The model under review builds one solid part; all positions refer to its coordinate system, in mm. A direction names the side the tool comes from. Give positions to 0.01 mm unless a question says otherwise; leave off trailing zeros. Write each loop counter-clockwise with the first axis right and the second up, starting at its lowest first coordinate (ties: lowest second). Pieces come first, ordered by that corner, then holes. Notation, with made-up numbers: (50.5, 89) - (93.5, 89) arc R15 cw to (93.5, 107) - close; hole circle Ø11 at (67, 67). An arc over 180 degrees is marked (long way). Write item = value, one per line.
```python
from build123d import *

# Parameters (mm, degrees)
EXTRUDE_1_DEPTH = 5


with BuildPart() as part:
    # 草图1 → 凸台-拉伸1 (new body)
    with BuildSketch(Plane.XY):
        with BuildLine():
            Line((36.5, -9.5), (36.5, 9.5))
            ThreePointArc((36.5, 9.5), (35.621320344, 11.621320344), (33.5, 12.5))
            Line((33.5, 12.5), (-33.5, 12.5))
            ThreePointArc((-33.5, 12.5), (-35.621320344, 11.621320344), (-36.5, 9.5))
            Line((-36.5, 9.5), (-36.5, -9.5))
            ThreePointArc((-36.5, -9.5), (-35.621320344, -11.621320344), (-33.5, -12.5))
            Line((-33.5, -12.5), (-2.5, -12.5))
            Line((-2.5, -12.5), (-2.5, 2.5))
            Line((-2.5, 2.5), (2.5, 2.5))
            Line((2.5, 2.5), (2.5, -12.5))
            Line((2.5, -12.5), (33.5, -12.5))
            ThreePointArc((33.5, -12.5), (35.621320344, -11.621320344), (36.5, -9.5))
        make_face()
        with BuildLine():
            Line((-19.75, -2.5), (-19.75, 6))
            ThreePointArc((-19.75, 6), (-16.5, 9.25), (-13.25, 6))
            Line((-13.25, 6), (-13.25, -2.5))
            ThreePointArc((-13.25, -2.5), (-16.5, -5.75), (-19.75, -2.5))
        make_face(mode=Mode.SUBTRACT)
        with BuildLine():
            Line((19.75, -2.5), (19.75, 6))
            ThreePointArc((19.75, 6), (16.5, 9.25), (13.25, 6))
            Line((13.25, 6), (13.25, -2.5))
            ThreePointArc((13.25, -2.5), (16.5, -5.75), (19.75, -2.5))
        make_face(mode=Mode.SUBTRACT)
    extrude(amount=EXTRUDE_1_DEPTH)


solid = part.part
```
1. Take a section at A-A on x = -16.5. Give the boundary of the cut face in (y, z), and give its area (3 significant figures).
Findings below:
outline = (-12.5, 0) - (-5.75, 0) - (-5.75, 5) - (-12.5, 5) - close; (9.25, 0) - (12.5, 0) - (12.5, 5) - (9.25, 5) - close
area = 50.0 mm²
2. Insertion check: P1, Ø3, axis at x = -7.5, y = 6, coming from the -Z side. The pin has a flat end and moves straight along its axis. Give the tip position at first contact, or say it passes through.
Findings below:
P1 = 0
3. For line 1 (X direction, y = 6.25, z = 4.65); line 2 (X direction, y = 4.25, z = 3.4); line 3 (X direction, y = -1.5, z = 3.6), list the stretches that pass through material, from the lowest coordinate up. Write a range as from..to.
Findings below:
line_1 = -36.5..-19.74, -13.26..13.26, 19.74..36.5
line_2 = -36.5..-19.75, -13.25..13.25, 19.75..36.5
line_3 = -36.5..-19.75, -13.25..-2.5, 2.5..13.25, 19.75..36.5
4. Draft analysis for pull direction Y (two halves, no side actions). For faces 1 (the flat face through (-13.25, 2, 2)), 2 (the flat face through (-36.5, 0, 2)), 3 (the flat face through (-18, -12.5, 2)), state which applies: +Y half, -Y half, draft (parallel to the pull), parting line (faces both ways), or undercut.
Findings below:
face_1 = undercut
face_2 = draft
face_3 = -Y half
5. Take a section at C-C on z = 1.35. Give the boundary of the cut face in (x, y).
Findings below:
outline = (-36.5, -9.5) arc R3 ccw to (-33.5, -12.5) - (-2.5, -12.5) - (-2.5, 2.5) - (2.5, 2.5) - (2.5, -12.5) - (33.5, -12.5) arc R3 ccw to (36.5, -9.5) - (36.5, 9.5) arc R3 ccw to (33.5, 12.5) - (-33.5, 12.5) arc R3 ccw to (-36.5, 9.5) - close; hole (-19.75, -2.5) arc R3.25 ccw to (-13.25, -2.5) - (-13.25, 6) arc R3.25 ccw to (-19.75, 6) - close; hole (13.25, -2.5) arc R3.25 ccw to (19.75, -2.5) - (19.75, 6) arc R3.25 ccw to (13.25, 6) - close
6. Machinability: for faces 4 (the cylindrical face through (35.64, 11.6, 2.46)), 5 (the cylindrical face through (-16.57, 9.25, 2.46)), 6 (the flat face through (2.5, -5, 2)), which of the approach directions +Z, -Z, +X, -X, +Y, -Y give a long, thin tool a straight path to every point of the face, cutting with its end or side? Answer none if there is none.
Findings below:
face_4 = +Z, -Z, +X, +Y
face_5 = +Z, -Z
face_6 = +Z, -Z, -Y
7. Take a section at B-B on y = -4.5. Give the boundary of the cut face in (x, z).
Findings below:
outline = (-36.5, 0) - (-19.06, 0) - (-19.06, 5) - (-36.5, 5) - close; (-13.94, 0) - (-2.5, 0) - (-2.5, 5) - (-13.94, 5) - close; (2.5, 0) - (13.94, 0) - (13.94, 5) - (2.5, 5) - close; (19.06, 0) - (36.5, 0) - (36.5, 5) - (19.06, 5) - close
